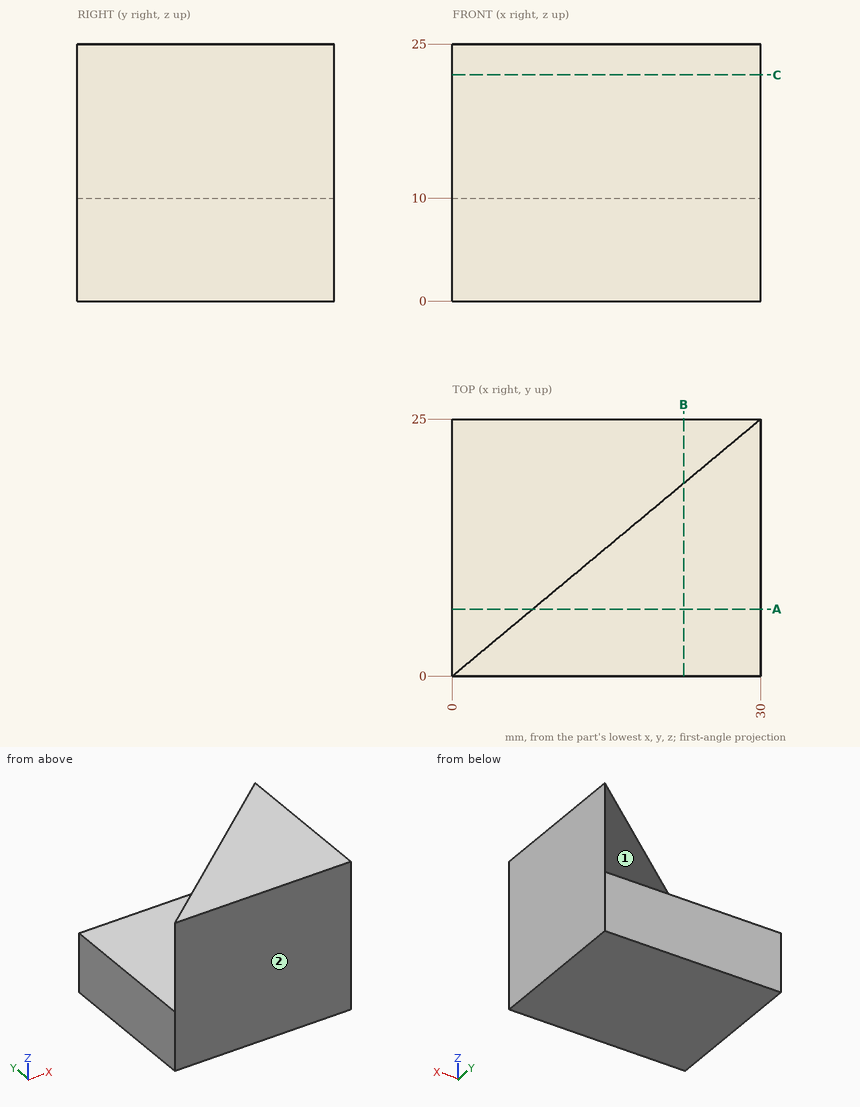
The drawing under review shows one solid part. Ordinate dimensions are in mm from its lowest x, y, z. A direction names the side the tool comes from. Round coordinates to 2 decimals unless told otherwise and drop trailing zeros. Order: outer loops, then holes, each group sorted by start corner. A loop starts at its lowest first (then second) coordinate and runs counter-clockwise, first axis right, second up. Notation, with made-up numbers: (29, 35) -> (78, 35) arc R25 ccw to (78, 50) -> close; hole circle Ø3 at (20, 27). An arc over 180 degrees is marked (long way). Use a Markdown table: item, result.
Item 1: Take a section at B-B (x = 22.5). State the section outline as (y, z) points, plus the area to 3 significant figures.
Resolved:
| item | result |
|---|---|
| outline | (0, 0) -> (25, 0) -> (25, 10) -> (18.75, 10) -> (18.75, 25) -> (0, 25) -> close |
| area | 531 mm² |
Item 2: For line 1 along Z through (x, y) = (3, 21.25); line 2 along Y through (x, z) = (27.75, 13.5) (3 decimals); line 3 along Y through (x, z) = (16.75, 19), list the stretches that pass through material, from the lowest coordinate up. Write a range as [from, to].
Resolved:
| item | result |
|---|---|
| line 1 | z = [0, 10] |
| line 2 | y = [0, 23.125] |
| line 3 | y = [0, 13.96] |
Item 3: Machinability: for the marked faces 1 and 2, which of the approach directions +Z, -Z, +X, -X, +Y, -Y give a long, thin tool a straight path to every point of the face, cutting with its end or side? Answer none if there is none.
Resolved:
| item | result |
|---|---|
| face 1 | +Z, -X, +Y |
| face 2 | +Z, -Z, +X, -X, -Y |
Item 4: Take a section at C-C (z = 22). State the section outline as (x, y) points.
Resolved:
| item | result |
|---|---|
| outline | (0, 0) -> (30, 0) -> (30, 25) -> close |
Item 5: For pin 1 (1 mm diameter, centred on x = 24.5, z = 20.5, fed in from +Y); pin 2 (4 mm diameter, centred on x = 16.5, z = 19, fed in from +Y), all flat-tipped, find the tip position at first contact; note any pin that passes through.
Resolved:
| item | result |
|---|---|
| pin 1 | stops at y = 20.83 |
| pin 2 | stops at y = 15.42 |
Item 6: Take a section at A-A (y = 6.5). State the section outline as (x, z) points.
Resolved:
| item | result |
|---|---|
| outline | (0, 0) -> (30, 0) -> (30, 25) -> (7.8, 25) -> (7.8, 10) -> (0, 10) -> close |
